Check sheet for the modelled part. Datum: model origin and axes. Units: mm. Round coordinates to 2 decimals unless told otherwise and drop trailing zeros. Write each loop counter-clockwise with the first axis right and the second up, starting at its lowest first coordinate (ties: lowest second). Pieces come first, ordered by that corner, then holes.
Item 1: Cross-section at B-B on z = 3.25. Count the separate pieces of the cut face and the enclosed holes in it, plus the area to 3 significant figures.
Item 2: Cross-section at A-A on y = 51. Enter the section's corners in (x, z), plus the area to 3 significant figures.
Item 3: Cross-section at D-D on y = -144.5. Enter the section's corners in (x, z), plus the area to 3 significant figures.
Item 4: Go/stop test with flat-tipped pins: pin 1 Ø4 at (x, z) = (3, 4) entering from +Y (3 decimals); pin 2 Ø4 at (x, z) = (-70, 6.5) entering from +Y; pin 3 Ø4 at (y, z) = (-191.5, 7.5) entering from -X; pin 4 Ø6 at (x, y) = (403.22, -80.93) entering from +Z. Record where each tip stops, or that it passes through.
Item 5: Cross-section at C-C on x = 200.5. Enter the section's corners in (y, z), plus the area to 3 significant figures.
Item 6: Material ranges on line 1 (X direction, y = 269.5, z = 3.5); line 2 (X direction, y = 95, z = 6.75); line 3 (Y direction, x = -2, z = 11.5) (3 decimals), recorded low to high.
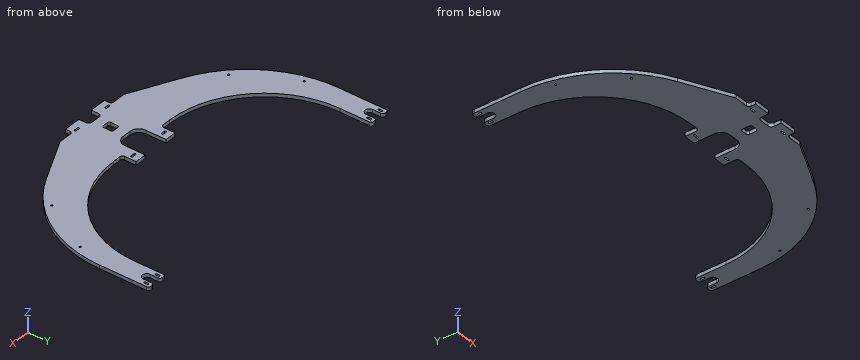
from build123d import *

# Parameters (mm, degrees)
BOSS_EXTRUDE1_DEPTH          = 12.7
CUT_EXTRUDE1_DEPTH           = 666.993618588
G_0_261_DIAMETER_SLOT1_DEPTH = 12.7
G_0_261_DIAMETER_SLOT2_DEPTH = 12.7
FILLET1_R                    = 9.525
SKETCH9_W                    = 57.15
SKETCH9_H                    = 38.1
CUT_EXTRUDE2_DEPTH           = 666.993618588
FILLET3_R                    = 12.7
SKETCH10_W                   = 95.25
SKETCH10_H                   = 104.775
CUT_EXTRUDE3_DEPTH           = 666.993618588
FILLET4_R                    = 31.75
F_1_4_CLEARANCE_HOLE1_D      = 6.7564
SKETCH13_W                   = 31.75
SKETCH13_H                   = 38.1
CUT_EXTRUDE4_DEPTH           = 666.993618588
FILLET5_R                    = 6.35


# Read off the part's stored shape, not the designer's step: G (0.261) Diameter Slot1, G (0.261) Diameter Slot2
with BuildPart() as part:
    # Sketch2 → Boss-Extrude1 (new body)
    with BuildSketch(Plane.XY):
        with BuildLine():
            Line((-88.9, -254), (-88.9, -279.4))
            Line((-88.9, -279.4), (88.9, -279.4))
            Line((88.9, -279.4), (88.9, -254))
            Line((88.9, -254), (146.05, -254))
            Line((146.05, -254), (311.089942486, -173.30458573))
            ThreePointArc((311.089942486, -173.30458573), (482.525600271, -18.715203517), (546.1, 203.2))
            Line((546.1, 203.2), (546.1, 304.8))
            Line((546.1, 304.8), (546.1, 381))
            Line((546.1, 381), (469.9, 381))
            Line((469.9, 381), (469.9, 304.8))
            Line((469.9, 304.8), (469.9, 266.7))
            ThreePointArc((469.9, 266.7), (369.466915269, 24.233084731), (127, -76.2))
            Line((127, -76.2), (88.9, -76.2))
            Line((88.9, -76.2), (88.9, -25.4))
            Line((88.9, -25.4), (-88.9, -25.4))
            Line((-88.9, -25.4), (-88.9, -76.2))
            Line((-88.9, -76.2), (-127, -76.2))
            ThreePointArc((-127, -76.2), (-369.466915269, 24.233084731), (-469.9, 266.7))
            Line((-469.9, 266.7), (-469.9, 304.8))
            Line((-469.9, 304.8), (-469.9, 381))
            Line((-469.9, 381), (-546.1, 381))
            Line((-546.1, 381), (-546.1, 304.8))
            Line((-546.1, 304.8), (-546.1, 203.2))
            ThreePointArc((-546.1, 203.2), (-482.525600271, -18.715203517), (-311.089942486, -173.30458573))
            Line((-311.089942486, -173.30458573), (-146.05, -254))
            Line((-146.05, -254), (-88.9, -254))
        make_face()
    extrude(amount=BOSS_EXTRUDE1_DEPTH)

    # Sketch3 → Cut-Extrude1 (cut, through all)
    with BuildSketch(Plane.XY.offset(12.7)):
        with BuildLine():
            Line((-523.0876, 342.9), (-523.0876, 381))
            Line((-523.0876, 381), (-492.9124, 381))
            Line((-492.9124, 381), (-492.9124, 342.9))
            ThreePointArc((-492.9124, 342.9), (-508, 327.8124), (-523.0876, 342.9))
        make_face()
        with BuildLine():
            Line((492.9124, 342.9), (492.9124, 381))
            Line((492.9124, 381), (523.0876, 381))
            Line((523.0876, 381), (523.0876, 342.9))
            ThreePointArc((523.0876, 342.9), (508, 327.8124), (492.9124, 342.9))
        make_face()
    extrude(amount=-CUT_EXTRUDE1_DEPTH, mode=Mode.SUBTRACT)

    # G (0.261) Diameter Slot1 outline → G (0.261) Diameter Slot1 (cut)
    with BuildSketch(Plane.XY):
        with BuildLine():
            ThreePointArc((-63.5, -257.3147), (-60.1853, -254), (-63.5, -250.6853))
            Line((-63.5, -250.6853), (-76.2, -250.6853))
            ThreePointArc((-76.2, -250.6853), (-79.5147, -254), (-76.2, -257.3147))
            Line((-76.2, -257.3147), (-63.5, -257.3147))
        make_face()
        with BuildLine():
            ThreePointArc((63.5, -250.6853), (60.1853, -254), (63.5, -257.3147))
            Line((63.5, -257.3147), (76.2, -257.3147))
            ThreePointArc((76.2, -257.3147), (79.5147, -254), (76.2, -250.6853))
            Line((76.2, -250.6853), (63.5, -250.6853))
        make_face()
        with BuildLine():
            ThreePointArc((-63.5, -54.1147), (-60.1853, -50.8), (-63.5, -47.4853))
            Line((-63.5, -47.4853), (-76.2, -47.4853))
            ThreePointArc((-76.2, -47.4853), (-79.5147, -50.8), (-76.2, -54.1147))
            Line((-76.2, -54.1147), (-63.5, -54.1147))
        make_face()
        with BuildLine():
            ThreePointArc((63.5, -47.4853), (60.1853, -50.8), (63.5, -54.1147))
            Line((63.5, -54.1147), (76.2, -54.1147))
            ThreePointArc((76.2, -54.1147), (79.5147, -50.8), (76.2, -47.4853))
            Line((76.2, -47.4853), (63.5, -47.4853))
        make_face()
    extrude(amount=G_0_261_DIAMETER_SLOT1_DEPTH, mode=Mode.SUBTRACT)

    # G (0.261) Diameter Slot2 outline → G (0.261) Diameter Slot2 (cut)
    with BuildSketch(Plane.XY):
        with BuildLine():
            ThreePointArc((-479.2853, 366.7125), (-482.6, 370.0272), (-485.9147, 366.7125))
            Line((-485.9147, 366.7125), (-485.9147, 357.1875))
            ThreePointArc((-485.9147, 357.1875), (-482.6, 353.8728), (-479.2853, 357.1875))
            Line((-479.2853, 357.1875), (-479.2853, 366.7125))
        make_face()
        with BuildLine():
            ThreePointArc((-530.0853, 366.7125), (-533.4, 370.0272), (-536.7147, 366.7125))
            Line((-536.7147, 366.7125), (-536.7147, 357.1875))
            ThreePointArc((-536.7147, 357.1875), (-533.4, 353.8728), (-530.0853, 357.1875))
            Line((-530.0853, 357.1875), (-530.0853, 366.7125))
        make_face()
        with BuildLine():
            ThreePointArc((485.9147, 366.7125), (482.6, 370.0272), (479.2853, 366.7125))
            Line((479.2853, 366.7125), (479.2853, 357.1875))
            ThreePointArc((479.2853, 357.1875), (482.6, 353.8728), (485.9147, 357.1875))
            Line((485.9147, 357.1875), (485.9147, 366.7125))
        make_face()
        with BuildLine():
            ThreePointArc((536.7147, 366.7125), (533.4, 370.0272), (530.0853, 366.7125))
            Line((530.0853, 366.7125), (530.0853, 357.1875))
            ThreePointArc((530.0853, 357.1875), (533.4, 353.8728), (536.7147, 357.1875))
            Line((536.7147, 357.1875), (536.7147, 366.7125))
        make_face()
    extrude(amount=G_0_261_DIAMETER_SLOT2_DEPTH, mode=Mode.SUBTRACT)

    # Fillet1
    fillet1_edges = [part.edges().sort_by_distance(p)[0] for p in [
        (469.9, 381, 6.35),
        (546.1, 381, 6.35),
        (146.05, -254, 6.35),
        (88.9, -254, 6.35),
        (-88.9, -254, 6.35),
        (-146.05, -254, 6.35),
        (-546.1, 381, 6.35),
        (-469.9, 381, 6.35),
        (-88.9, -76.2, 6.35),
        (88.9, -76.2, 6.35),
        (492.9124, 381, 6.35),
        (523.0876, 381, 6.35),
        (-523.0876, 381, 6.35),
        (-492.9124, 381, 6.35),
    ]]
    fillet(fillet1_edges, radius=FILLET1_R)

    # Sketch9 → Cut-Extrude2 (cut, through all)
    with BuildSketch(Plane.XY.offset(12.7)):
        with Locations((0, -260.35)):
            Rectangle(SKETCH9_W, SKETCH9_H)
    extrude(amount=-CUT_EXTRUDE2_DEPTH, mode=Mode.SUBTRACT)

    # Fillet3
    fillet3_edges = [part.edges().sort_by_distance(p)[0] for p in [
        (-28.575, -241.3, 6.35),
        (28.575, -241.3, 6.35),
    ]]
    fillet(fillet3_edges, radius=FILLET3_R)

    # Sketch10 → Cut-Extrude3 (cut, through all)
    with BuildSketch(Plane.XY.offset(12.7)):
        with Locations((0, -77.7875)):
            Rectangle(SKETCH10_W, SKETCH10_H)
    extrude(amount=-CUT_EXTRUDE3_DEPTH, mode=Mode.SUBTRACT)

    # Fillet4
    fillet4_edges = [part.edges().sort_by_distance(p)[0] for p in [
        (-47.625, -130.175, 6.35),
        (47.625, -130.175, 6.35),
    ]]
    fillet(fillet4_edges, radius=FILLET4_R)

    # 1/4 Clearance Hole1 (through all)
    with Locations(Plane.XY.offset(12.7)):
        with Locations((403.225, -80.928501225), (511.175, 106.046383452)):
            f_1_4_clearance_hole1 = Hole(F_1_4_CLEARANCE_HOLE1_D / 2)

    # Mirror1: 1/4 Clearance Hole1 across plane
    add(f_1_4_clearance_hole1.mirror(Plane(origin=(0, 0, 0), x_dir=(0, 0, 1), z_dir=(1, 0, 0))), mode=Mode.SUBTRACT)

    # Sketch13 → Cut-Extrude4 (cut, through all)
    with BuildSketch(Plane.XY.offset(12.7)):
        with Locations((0, -187.325)):
            Rectangle(SKETCH13_W, SKETCH13_H)
    extrude(amount=-CUT_EXTRUDE4_DEPTH, mode=Mode.SUBTRACT)

    # Fillet5
    fillet5_edges = [part.edges().sort_by_distance(p)[0] for p in [
        (15.875, -168.275, 6.35),
        (15.875, -206.375, 6.35),
        (-15.875, -206.375, 6.35),
        (-15.875, -168.275, 6.35),
    ]]
    fillet(fillet5_edges, radius=FILLET5_R)


solid = part.part
Response values:
1. separate pieces: 1
1. enclosed holes: 13
1. area: 209,000 mm2
2. outline: (-517.49, 0) - (-393.56, 0) - (-393.56, 12.7) - (-517.49, 12.7) - close; (393.56, 0) - (517.49, 0) - (517.49, 12.7) - (393.56, 12.7) - close
2. area: 3,150 mm2
3. outline: (-360.99, 0) - (360.99, 0) - (360.99, 12.7) - (-360.99, 12.7) - close
3. area: 9,170 mm2
4. pin 1: stops at y = -130.175
4. pin 2: stops at y = -25.4
4. pin 3: stops at x = -277.97
4. pin 4: passes through
5. outline: (-227.38, 0) - (-68.23, 0) - (-68.23, 12.7) - (-227.38, 12.7) - close
5. area: 2,020 mm2
6. line 1: x = -546.1 to -469.9, 469.9 to 546.1
6. line 2: x = -531.89 to -423.82, 423.82 to 531.89
6. line 3: y = -241.3 to -206.375, -168.275 to -130.175
